Here's how the part is built. I have some questions about the finished solid (model axes, mm). A direction names the side the tool comes from. Round coordinates to 2 decimals unless told otherwise and drop trailing zeros. Loops run counter-clockwise (first coordinate to the right, second up) from the corner with the lowest first, then second, coordinate; pieces in that order, holes last. Notation, with made-up numbers: M -12,15 L 24,15 A17 cw 24,39 Z; hole C 6.5,66 d6. An arc over 180 degrees is marked long. Answer as CSV lines item,"result".
Autodesk Inventor part; units mm, degrees
ref_plane "Plano de trabajo14" through (0, 0, 40) normal (0, 0, 1) x (1, 0, 0)
ref_plane "Plano de trabajo15" through (0, 0, 40) normal (0, 0, -1) x (-1, 0, 0)
ref_plane "YZ Plane" through (0, 0, 0) normal (1, 0, 0) x (0, 1, 0)
ref_plane "Plano de trabajo14" through (0, 0, 40) normal (0, 0, 1) x (1, 0, 0)
sketch "Boceto6" plane through (0, 0, 40) normal (0, 0, 1) x (1, 0, 0)
  line L0 (49.7736, 62.508) -> (29.5128, 46.2994)
  line L1 (28.7888, 42.4568) -> (29.4835, 41.2536)
  line L2 (47.1158, -3.8365) -> (27.2606, -8.2224)
  arc A0 (29.5128, 46.2994) -> (28.7888, 42.4568) centre (31.3869, 43.9568) ccw
  arc A1 (29.8562, 39.3361) -> (29.4835, 41.2536) centre (26.8854, 39.7536) ccw
  arc A2 (54.2458, 61.6654) -> (49.7736, 62.508) centre (51.6477, 60.1654) ccw
  arc A3 (23.6427, -4.8755) -> (27.2606, -8.2224) centre (26.6135, -5.293) ccw
  arc A4 (47.1158, -3.8365) -> (49.4395, -1.3246) centre (46.4687, -0.9071) ccw
  arc A5 (57.2604, 54.324) -> (56.6392, 57.5198) centre (52.3091, 55.0198) ccw
  arc A6 (56.6392, 57.5198) -> (54.2458, 61.6654) centre (47.0339, 54.7379) ccw
  arc A7 (49.4395, -1.3246) -> (57.2604, 54.324) centre (-341.7788, 82.0314) ccw
  arc A8 (23.6427, -4.8755) -> (29.8562, 39.3361) centre (-368.7404, 72.8128) ccw
  line L3 (51.5494, 60.0868) -> (31.3869, 43.9568)
  line L4 (31.3869, 43.9568) -> (32.0816, 42.7536)
  arc A9 (32.8399, 39.0157) -> (32.0816, 42.7536) centre (26.8854, 39.7536) ccw
  arc A10 (26.6185, -5.2919) -> (32.8399, 39.0157) centre (-368.7404, 72.8128) ccw
  line L5 (26.6185, -5.2919) -> (46.4607, -0.9089)
  arc A11 (46.4607, -0.9089) -> (54.2765, 54.6606) centre (-341.7788, 82.0314) ccw
  arc A12 (54.2765, 54.6606) -> (53.8619, 56.2803) centre (52.3091, 55.0198) ccw
  arc A13 (53.8619, 56.2803) -> (51.5494, 60.0868) centre (47.0339, 54.7379) ccw
  dimension "d106" = 3
extrude "Extrusión11" add sketch "Boceto6" against normal blind 2 contours A2 A6 A5 A7 A4 L2 A3 A8 A1 L1 A0 L0 | A13 A12 A11 L5 A10 A9 L4 L3
ref_plane "Plano de trabajo15" through (0, 0, 40) normal (0, 0, -1) x (-1, 0, 0)
sketch "Boceto34" plane through (0, 0, 40) normal (0, 0, 1) x (1, 0, 0)
  line L0 (47.4839, 60.6763) -> (33.5541, 49.5324)
  line L1 (39.6432, 54.4037) -> (42.1142, 54.4037) construction
  line L2 (39.6432, 54.4037) -> (42.3572, 54.4037) construction
  arc A0 (33.5541, 49.5324) -> (47.4839, 60.6763) centre (38.9752, 57.0342) ccw
  point P0 (0, 0)
  dimension "d154" = 18.511
extrude "Extrusión26" cut sketch "Boceto34" against normal blind 10
equation "\"Radio_pliegue\" = Grosor"
equation "\"Anchura_desahogo_plegado\" = Grosor"
equation "\"Profundidad_desahogo_plegado\" = 0.5 * Grosor"
equation "\"Tamaño_destalonado\" = 4 * Grosor"
equation "\"Remanente_mínimo\" = 2 * Grosor"
equation "\"Radiodetransición\" = Radio_pliegue"
equation "\"Tamaño_de_radio_de_Jacobi\" = Radio_pliegue"
equation "\"TamañoSeparación\" = Grosor"
properties part number "brazocuadrado"
1. If I drill on line 1 (X direction, y = 15.5, z = 39.95); line 2 (Y direction, x = 46.5, z = 38.45); line 3 (X direction, y = 8, z = 38.6), over which ranges is the centre line in solid material (lowest first)? Write a range as [from, to].
Evaluation:
line 1,"x = [27.13, 52.65]"
line 2,"y = [-3.97, 51.65]"
line 3,"x = [25.97, 51.31]"
2. We'd pull the mould along Y, two halves only. Please class faces 3 (the cylindrical face through (54.273, 25.972, 39.014)), 4 (the flat face through (40, 28, 40)), 5 (the cylindrical face through (28.444, 44.542, 39.014)): pulls with the +Y half, pulls with the -Y half, needs draft (parallel to the pull), parting line crosses it, or undercut.
Evaluation:
face 3,"pulls with the -Y half"
face 4,"needs draft"
face 5,"undercut"
3. For P1, Ø1, axis at y = 20, z = 38, coming from the +X side, with a flat end and sliding along its axis, tell me the tip position at first contact or that it passes through.
Evaluation:
P1,"stops at x = 53.46"
4. I want a section at B-B, the plane y = 52.5. Please give me the cut outline in (x, z), and give its area (3 significant figures).
Evaluation:
outline,"M 47.04,38 L 57.13,38 L 57.13,40 L 47.04,40 Z"
area,"20.2 mm²"
5. I want a section at C-C, the plane x = 32.5. Please give me the cut outline in (y, z), and give its area (3 significant figures).
Evaluation:
outline,"M -7.07,38 L 48.69,38 L 48.69,40 L -7.07,40 Z"
area,"112 mm²"
6. Which directions (+Z, -Z, +X, -X, +Y, -Y) give clear straight access to the entire face, cutting with the end or side of a thin tool? Please do faces 1 (the flat face through (29.131, 41.864, 39.014)), 2 (the flat face through (31.562, 47.939, 39.014)).
Evaluation:
face 1,"+Z, -Z, -X"
face 2,"+Z, -Z, -X, +Y"
7. I want a section at A-A, the plane z = 39.05. Please give me the cut outline in (x, y).
Evaluation:
outline,"M 23.64,-4.88 A3 ccw 27.26,-8.22 L 47.12,-3.84 A3 ccw 49.44,-1.32 A400 ccw 57.26,54.32 A5 ccw 56.64,57.52 A10 ccw 54.25,61.67 A3 ccw 49.77,62.51 L 47.48,60.68 A9.26 cw 33.55,49.53 L 29.51,46.3 A3 ccw 28.79,42.46 L 29.48,41.25 A3 cw 29.86,39.34 A399.99 cw Z"
